from build123d import *

# Parameters (mm, degrees)
SKETCH_1_R          = 1.7
SKETCH_1_W          = 5
SKETCH_1_H          = 13
SKETCH_1_H_2        = 2
EXTRUDE_3_DEPTH     = 2.9
SKETCH_3_R          = 2.1
CUT_EXTRUDE_3_DEPTH = 2.9
SKETCH_4_W          = 20
SKETCH_4_H          = 40
SKETCH_4_R          = 2.1
EXTRUDE_4_DEPTH     = 2.9
SKETCH_5_W          = 70
SKETCH_5_H          = 40
SKETCH_5_W_2        = 69.6
SKETCH_5_H_2        = 39.6
CUT_EXTRUDE_4_DEPTH = 2.9
SKETCH_6_W          = 9.917430794
SKETCH_6_H          = 39.6
SKETCH_6_R          = 2.1
CUT_EXTRUDE_5_DEPTH = 10


with BuildPart() as part:
    # 草图1 → 凸台-拉伸3 (new body)
    # profile 1 of 10: a face of its own
    with BuildSketch(Plane(origin=(0, 0, 0), x_dir=(1, 0, 0), z_dir=(0, 1, 0))):
        with BuildLine():
            Line((-40, 113), (-70, 113))
            Line((-70, 113), (-70, 108))
            Line((-70, 108), (-70, 92))
            Line((-70, 92), (-63.7, 92))
            ThreePointArc((-63.7, 92), (-62, 93.7), (-60.3, 92))
            ThreePointArc((-60.3, 92), (-60.797918472, 90.797918472), (-62, 90.3))
            Line((-62, 90.3), (-62, 87))
            Line((-62, 87), (-48, 87))
            Line((-48, 87), (-48, 90.3))
            ThreePointArc((-48, 90.3), (-49.202081528, 93.202081528), (-46.3, 92))
            Line((-46.3, 92), (-40, 92))
            Line((-40, 92), (-40, 113))
        make_face()
        with Locations(Location((-62, 108, 0), (0, 0, 270))):
            Circle(SKETCH_1_R, mode=Mode.SUBTRACT)
        with Locations(Location((-48, 108, 0), (0, 0, 270))):
            Circle(SKETCH_1_R, mode=Mode.SUBTRACT)
    # profile 2 of 10: a face of its own
    with BuildSketch(Plane(origin=(0, 0, 0), x_dir=(1, 0, 0), z_dir=(0, 1, 0))):
        with BuildLine():
            Line((-70, 92), (-70, 87))
            Line((-70, 87), (-62, 87))
            Line((-62, 87), (-62, 90.3))
            ThreePointArc((-62, 90.3), (-63.202081528, 90.797918472), (-63.7, 92))
            Line((-63.7, 92), (-70, 92))
        make_face()
    # profile 3 of 10: a face of its own
    with BuildSketch(Plane(origin=(0, 0, 0), x_dir=(1, 0, 0), z_dir=(0, 1, 0))):
        with BuildLine():
            Line((-48, 90.3), (-48, 87))
            Line((-48, 87), (-40, 87))
            Line((-40, 87), (-40, 92))
            Line((-40, 92), (-46.3, 92))
            ThreePointArc((-46.3, 92), (-46.797918472, 90.797918472), (-48, 90.3))
        make_face()
    # profile 4 of 10: a face of its own
    with BuildSketch(Plane(origin=(0, 0, 0), x_dir=(1, 0, 0), z_dir=(0, 1, 0))):
        Polygon((-70, 87), (-70, 80), (-20, 80), (-20, 85), (-25, 85), (-25, 87), (-40, 87), (-48, 87), (-62, 87), align=None)
    # profile 5 of 10: a face of its own
    with BuildSketch(Plane(origin=(0, 0, 0), x_dir=(1, 0, 0), z_dir=(0, 1, 0))):
        Polygon((-25, 113), (-40, 113), (-40, 92), (-40, 87), (-25, 87), (-25, 100), align=None)
    # profile 6 of 10: a face of its own
    with BuildSketch(Plane(origin=(0, 0, 0), x_dir=(1, 0, 0), z_dir=(0, 1, 0))):
        with Locations((-22.5, 93.5)):
            Rectangle(SKETCH_1_W, SKETCH_1_H)
    # profile 7 of 10: a face of its own
    with BuildSketch(Plane(origin=(0, 0, 0), x_dir=(1, 0, 0), z_dir=(0, 1, 0))):
        with Locations((-22.5, 106.5)):
            Rectangle(SKETCH_1_W, SKETCH_1_H)
    # profile 8 of 10: a face of its own
    with BuildSketch(Plane(origin=(0, 0, 0), x_dir=(1, 0, 0), z_dir=(0, 1, 0))):
        with Locations((-22.5, 86)):
            Rectangle(SKETCH_1_W, SKETCH_1_H_2)
    # profile 9 of 10: a face of its own
    with BuildSketch(Plane(origin=(0, 0, 0), x_dir=(1, 0, 0), z_dir=(0, 1, 0))):
        Polygon((-20, 120), (-70, 120), (-70, 113), (-40, 113), (-25, 113), (-25, 115), (-20, 115), align=None)
    # profile 10 of 10: a face of its own
    with BuildSketch(Plane(origin=(0, 0, 0), x_dir=(1, 0, 0), z_dir=(0, 1, 0))):
        with Locations((-22.5, 114)):
            Rectangle(SKETCH_1_W, SKETCH_1_H_2)
    extrude(amount=EXTRUDE_3_DEPTH)

    # 草图3 → 切除-拉伸3 (cut)
    with BuildSketch(Plane(origin=(0, 2.9, 0), x_dir=(1, 0, 0), z_dir=(0, 1, 0))):
        with Locations(Location((-25, 110, 0), (0, 0, 270))):
            Circle(SKETCH_3_R)
        with Locations(Location((-25, 90, 0), (0, 0, 270))):
            Circle(SKETCH_3_R)
        with Locations(Location((-35, 90, 0), (0, 0, 270))):
            Circle(SKETCH_3_R)
        with Locations(Location((-35, 110, 0), (0, 0, 270))):
            Circle(SKETCH_3_R)
    extrude(amount=-CUT_EXTRUDE_3_DEPTH, mode=Mode.SUBTRACT)

    # 草图4 → 凸台-拉伸4 (add)
    with BuildSketch(Plane(origin=(0, 2.9, 0), x_dir=(1, 0, 0), z_dir=(0, 1, 0))):
        with Locations((-10, 100)):
            Rectangle(SKETCH_4_W, SKETCH_4_H)
        with Locations(Location((-15, 110, 0), (0, 0, 270))):
            Circle(SKETCH_4_R, mode=Mode.SUBTRACT)
        with Locations(Location((-15, 90, 0), (0, 0, 270))):
            Circle(SKETCH_4_R, mode=Mode.SUBTRACT)
        with Locations(Location((-5, 110, 0), (0, 0, 270))):
            Circle(SKETCH_4_R, mode=Mode.SUBTRACT)
        with Locations(Location((-5, 90, 0), (0, 0, 270))):
            Circle(SKETCH_4_R, mode=Mode.SUBTRACT)
    extrude(amount=-EXTRUDE_4_DEPTH)

    # 草图5 → 切除-拉伸4 (cut)
    with BuildSketch(Plane(origin=(0, 2.9, 0), x_dir=(1, 0, 0), z_dir=(0, 1, 0))):
        with Locations((-35, 100)):
            Rectangle(SKETCH_5_W, SKETCH_5_H)
        with Locations((-35, 100)):
            Rectangle(SKETCH_5_W_2, SKETCH_5_H_2, mode=Mode.SUBTRACT)
    extrude(amount=-CUT_EXTRUDE_4_DEPTH, mode=Mode.SUBTRACT)

    # 草图6 → 切除-拉伸5 (cut)
    with BuildSketch(Plane(origin=(0, 2.9, 0), x_dir=(1, 0, 0), z_dir=(0, 1, 0))):
        with Locations((-5.158715397, 100)):
            Rectangle(SKETCH_6_W, SKETCH_6_H)
        with Locations((-5, 90)):
            Circle(SKETCH_6_R, mode=Mode.SUBTRACT)
        with Locations((-5, 110)):
            Circle(SKETCH_6_R, mode=Mode.SUBTRACT)
    extrude(amount=-CUT_EXTRUDE_5_DEPTH, mode=Mode.SUBTRACT)


solid = part.part
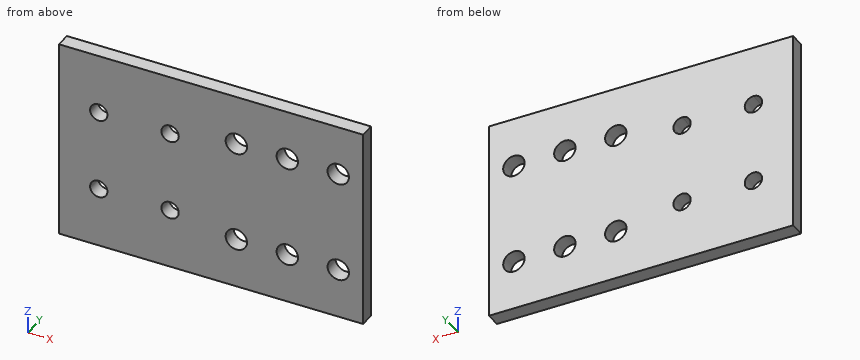
The listing builds one solid part. Answer for the finished solid, in the listing's coordinates (mm). Coordinates: 2 decimals unless noted, no trailing zeros. Write each loop counter-clockwise with the first axis right and the second up, starting at its lowest first coordinate (ties: lowest second). Pieces come first, ordered by that corner, then holes. Notation, with made-up numbers: (77.25, 14) - (93.25, 14) arc R16 cw to (93.25, 43) - close; hole circle Ø2 at (58.5, 64). An arc over 180 degrees is marked (long way). Return JSON: item names as keys, results as strings.
1. Consider line 1 along X through (y, z) = (0.6, -90); line 2 along Z through (x, y) = (-26.5, 1.4); line 3 along X through (y, z) = (0.65, -90.5). Determine where each line is inside the solid, lowest interval first.
Final values:
{"line 1": "-69.8 to -37.1, -32.9 to -27.1, -22.9 to -17.1, -12.9 to -10.12", "line 2": "-119.8 to -111.47, -108.53 to -91.47, -88.53 to -80.2", "line 3": "-69.8 to -62.8, -61.2 to -48.8, -47.2 to -37.04, -32.96 to -27.04, -22.96 to -17.04, -12.96 to -10.12"}
2. The part is cut by section A-A on x = -35. Determine the outline of the cut face in (y, z), then the cut area to 3 significant figures.
Final values:
{"outline": "(0, -119.8) - (2.9, -119.8) - (2.9, -112.1) - (0, -112.1) - close; (0, -107.9) - (2.9, -107.9) - (2.9, -92.1) - (0, -92.1) - close; (0, -87.9) - (2.9, -87.9) - (2.9, -80.2) - (0, -80.2) - close", "area": "90.5 mm^2"}
3. The part is cut by section C-C on z = -107. Determine the outline of the cut face in (x, y).
Final values:
{"outline": "(-69.8, 0) - (-63.37, 0) - (-63.37, 2.9) - (-69.8, 2.9) - close; (-60.63, 0) - (-49.37, 0) - (-49.37, 2.9) - (-60.63, 2.9) - close; (-46.63, 0) - (-10.12, 0) - (-10.12, 2.9) - (-46.63, 2.9) - close"}
4. The part is cut by section B-B on y = 1.9. Count the separate pieces of the cut face and the enclosed holes in it, then the cut area to 3 significant figures.
Final values:
{"separate pieces": "1", "enclosed holes": "10", "area": "2,240 mm^2"}
